Work out the finished part from the listing and answer in its coordinate system (mm). Give positions to 0.01 mm unless a question says otherwise; leave off trailing zeros. Loops run counter-clockwise (first coordinate to the right, second up) from the corner with the lowest first, then second, coordinate; pieces in that order, holes last. Notation, with made-up numbers: (16.25, -36) - (39.25, -36) arc R8 ccw to (39.25, -27) - close; hole circle Ø6 at (8, 4). An arc over 180 degrees is marked (long way). Use one line per item in the form item = value. Start each with the question number.
from build123d import *

# Parameters (mm, degrees)
SKETCH2_W           = 39
SKETCH2_H           = 39
SKETCH2_W_2         = 33
SKETCH2_H_2         = 33
BOSS_EXTRUDE1_DEPTH = 5
SKETCH1_R           = 0.95
CUT_EXTRUDE1_DEPTH  = 6


with BuildPart() as part:
    # Sketch2 → Boss-Extrude1 (new body)
    with BuildSketch(Plane(origin=(0, 0, 0), x_dir=(1, 0, 0), z_dir=(0, 1, 0))):
        Rectangle(SKETCH2_W, SKETCH2_H)
        Rectangle(SKETCH2_W_2, SKETCH2_H_2, mode=Mode.SUBTRACT)
    extrude(amount=BOSS_EXTRUDE1_DEPTH)

    # Sketch1 → Cut-Extrude1 (cut, through all)
    with BuildSketch(Plane(origin=(0, 0, 0), x_dir=(1, 0, 0), z_dir=(0, 1, 0))):
        with Locations((-17.909, -17.909)):
            Circle(SKETCH1_R)
        with Locations((-15.519, -17.909)):
            Circle(SKETCH1_R)
        with Locations((-13.129, -17.909)):
            Circle(SKETCH1_R)
        with Locations((-10.739, -17.909)):
            Circle(SKETCH1_R)
        with Locations((-8.349, -17.909)):
            Circle(SKETCH1_R)
        with Locations((-5.959, -17.909)):
            Circle(SKETCH1_R)
        with Locations((-3.569, -17.909)):
            Circle(SKETCH1_R)
        with Locations((-1.179, -17.909)):
            Circle(SKETCH1_R)
        with Locations((1.211, -17.909)):
            Circle(SKETCH1_R)
        with Locations((3.601, -17.909)):
            Circle(SKETCH1_R)
        with Locations((5.991, -17.909)):
            Circle(SKETCH1_R)
        with Locations((8.381, -17.909)):
            Circle(SKETCH1_R)
        with Locations((10.771, -17.909)):
            Circle(SKETCH1_R)
        with Locations((13.161, -17.909)):
            Circle(SKETCH1_R)
        with Locations((15.551, -17.909)):
            Circle(SKETCH1_R)
        with Locations((17.909, 17.909)):
            Circle(SKETCH1_R)
        with Locations((17.909, -17.941)):
            Circle(SKETCH1_R)
        with Locations((17.909, -15.551)):
            Circle(SKETCH1_R)
        with Locations((17.909, -13.161)):
            Circle(SKETCH1_R)
        with Locations((17.909, -10.771)):
            Circle(SKETCH1_R)
        with Locations((17.909, -8.381)):
            Circle(SKETCH1_R)
        with Locations((17.909, -5.991)):
            Circle(SKETCH1_R)
        with Locations((17.909, -3.601)):
            Circle(SKETCH1_R)
        with Locations((17.909, -1.211)):
            Circle(SKETCH1_R)
        with Locations((17.909, 1.179)):
            Circle(SKETCH1_R)
        with Locations((17.909, 3.569)):
            Circle(SKETCH1_R)
        with Locations((17.909, 5.959)):
            Circle(SKETCH1_R)
        with Locations((17.909, 8.349)):
            Circle(SKETCH1_R)
        with Locations((17.909, 10.739)):
            Circle(SKETCH1_R)
        with Locations((17.909, 13.129)):
            Circle(SKETCH1_R)
        with Locations((17.909, 15.519)):
            Circle(SKETCH1_R)
        with Locations((15.519, 17.909)):
            Circle(SKETCH1_R)
        with Locations((13.129, 17.909)):
            Circle(SKETCH1_R)
        with Locations((10.739, 17.909)):
            Circle(SKETCH1_R)
        with Locations((8.349, 17.909)):
            Circle(SKETCH1_R)
        with Locations((5.959, 17.909)):
            Circle(SKETCH1_R)
        with Locations((3.569, 17.909)):
            Circle(SKETCH1_R)
        with Locations((1.179, 17.909)):
            Circle(SKETCH1_R)
        with Locations((-1.211, 17.909)):
            Circle(SKETCH1_R)
        with Locations((-3.601, 17.909)):
            Circle(SKETCH1_R)
        with Locations((-5.991, 17.909)):
            Circle(SKETCH1_R)
        with Locations((-8.381, 17.909)):
            Circle(SKETCH1_R)
        with Locations((-10.771, 17.909)):
            Circle(SKETCH1_R)
        with Locations((-13.161, 17.909)):
            Circle(SKETCH1_R)
        with Locations((-15.551, 17.909)):
            Circle(SKETCH1_R)
        with Locations((-17.909, 17.941)):
            Circle(SKETCH1_R)
        with Locations((-17.909, 15.551)):
            Circle(SKETCH1_R)
        with Locations((-17.909, 13.161)):
            Circle(SKETCH1_R)
        with Locations((-17.909, 10.771)):
            Circle(SKETCH1_R)
        with Locations((-17.909, 8.381)):
            Circle(SKETCH1_R)
        with Locations((-17.909, 5.991)):
            Circle(SKETCH1_R)
        with Locations((-17.909, 3.601)):
            Circle(SKETCH1_R)
        with Locations((-17.909, 1.211)):
            Circle(SKETCH1_R)
        with Locations((-17.909, -1.179)):
            Circle(SKETCH1_R)
        with Locations((-17.909, -3.569)):
            Circle(SKETCH1_R)
        with Locations((-17.909, -5.959)):
            Circle(SKETCH1_R)
        with Locations((-17.909, -8.349)):
            Circle(SKETCH1_R)
        with Locations((-17.909, -10.739)):
            Circle(SKETCH1_R)
        with Locations((-17.909, -13.129)):
            Circle(SKETCH1_R)
        with Locations((-17.909, -15.519)):
            Circle(SKETCH1_R)
    extrude(amount=CUT_EXTRUDE1_DEPTH, mode=Mode.SUBTRACT)


solid = part.part
1) A cutting plane is placed at B-B (y = 2.1). State how many separate pieces and enclosed holes the cut face has, plus the area to 3 significant figures.
2) Determine the mould class of faces 1 (the flat face through (0, 2, -19.5)), 2 (the flat face through (-16.5, 2, 0)) for opening direction Z: released by +Z, released by -Z, zero draft, split by the parting line, or undercut.
3) A cutting plane is placed at A-A (x = -3.5). Give the vertices of the cut face in (y, z), plus the area to 3 significant figures.
4) Find the intervals of material crossed by probe 1 along Z at (x, y) = (6, 4.4); probe 2 along X at (y, z) = (1, -2), in increasing order.
Answer sheet:
q1.separate_pieces = 1
q1.enclosed_holes = 61
q1.area = 262 mm²
q2.face_1 = released by -Z
q2.face_2 = undercut
q3.outline = (0, -19.5) - (5, -19.5) - (5, -18.85) - (0, -18.85) - close; (0, -16.96) - (5, -16.96) - (5, -16.5) - (0, -16.5) - close; (0, 16.5) - (5, 16.5) - (5, 16.96) - (0, 16.96) - close; (0, 18.86) - (5, 18.86) - (5, 19.5) - (0, 19.5) - close
q3.area = 11.1 mm²
q4.probe_1 = -19.5 to -18.86, -16.96 to -16.5, 16.5 to 16.96, 18.86 to 19.5
q4.probe_2 = -19.5 to -18.44, -17.38 to -16.5, 16.5 to 17.43, 18.39 to 19.5
